Design review of the part built by this model. Coordinates are the model's own, in mm. A direction names the side the tool comes from. Coordinates: 2 decimals unless noted, no trailing zeros. Loops run counter-clockwise (first coordinate to the right, second up) from the corner with the lowest first, then second, coordinate; pieces in that order, holes last.
Autodesk Inventor part; units mm, degrees
ref_plane "YZ Plane" through (0, 0, 0) normal (1, 0, 0) x (0, 1, 0)
ref_plane "XZ Plane" through (0, 0, 0) normal (0, 1, 0) x (-1, 0, 0)
ref_plane "XY Plane" through (0, 0, 0) normal (0, 0, 1) x (1, 0, 0)
sketch "Sketch1" plane through (0, 0, 0) normal (0, 0, 1) x (1, 0, 0)
  line L0 (0, 0) -> (0, -50.8)
  line L1 (0, -50.8) -> (4, -50.8)
  line L2 (4, 0) -> (4, -50.8)
  line L3 (0, 0) -> (4, 0)
  line L4 (0, -63.5) -> (0, -72.2)
  line L5 (0, -72.2) -> (4, -72.2)
  line L6 (4, -63.5) -> (4, -72.2)
  line L7 (0, -63.5) -> (4, -63.5)
  line L8 (0, 21.4) -> (0, 12.7)
  line L9 (0, 12.7) -> (4, 12.7)
  line L10 (4, 21.4) -> (4, 12.7)
  line L11 (0, 21.4) -> (4, 21.4)
  line L12 (44.45, 25.4) -> (57.15, 25.4)
  line L13 (44.45, 25.4) -> (44.45, 21.4)
  line L14 (44.45, 21.4) -> (57.15, 21.4)
  line L15 (57.15, 25.4) -> (57.15, 21.4)
  line L16 (44.45, -76.2) -> (57.15, -76.2)
  line L17 (57.15, -76.2) -> (57.15, -72.2)
  line L18 (44.45, -72.2) -> (57.15, -72.2)
  line L19 (44.45, -76.2) -> (44.45, -72.2)
  line L20 (101.6, 21.4) -> (4, 21.4)
  line L21 (4, 21.4) -> (4, -72.2)
  line L22 (4, -72.2) -> (101.6, -72.2)
  line L23 (101.6, -72.2) -> (101.6, 21.4)
  line L24 (50.8, 21.4) -> (50.8, -72.2)
  line L25 (101.6, 0) -> (101.6, -50.8)
  line L26 (101.6, -50.8) -> (97.6, -50.8)
  line L27 (97.6, 0) -> (97.6, -50.8)
  line L28 (101.6, 0) -> (97.6, 0)
  line L29 (101.6, -63.5) -> (101.6, -72.2)
  line L30 (101.6, -72.2) -> (97.6, -72.2)
  line L31 (97.6, -63.5) -> (97.6, -72.2)
  line L32 (101.6, -63.5) -> (97.6, -63.5)
  line L33 (101.6, 21.4) -> (101.6, 12.7)
  line L34 (101.6, 12.7) -> (97.6, 12.7)
  line L35 (101.6, 21.4) -> (97.6, 21.4)
  line L36 (97.6, 12.7) -> (97.6, 21.4)
  line L37 (97.6, 12.7) -> (97.6, 0)
  line L38 (97.6, -50.8) -> (97.6, -63.5)
extrude "Extrusion1" add sketch "Sketch1" along normal blind 4 contours L3 L2 L1 L0 | L21 L10 L20 L14 L24 L18 L22 L6 L2 | L9 L8 L11 L10 | L6 L5 L4 L7 | L13 L12 L15 L14 | L18 L17 L16 L19 | L14 L20 L36 L37 L27 L38 L31 L22 L18 L24 | L20 L23 L34 L36 | L31 L32 L23 L22 | L28 L23 L26 L27
ref_plane "Work Plane1" through (50.8, -50.8, 0) normal (1, 0, 0) x (0, 0, -1)
sketch "Sketch2" plane through (0, 0, 4) normal (0, 0, 1) x (1, 0, 0)
  circle A0 centre (10.35, 6.35) radius 1.905
  line L0 (4, 12.7) -> (4, 0)
  point P0 (0, 0)
  point P1 (4, 6.35)
  point P2 (4, 6.35)
  dimension "d2" = 3.81
  dimension "d3" = 6.35
extrude "Extrusion2" cut sketch "Sketch2" against normal through all
properties part number "Left Panel" material "Wood (Cherry)"
Q1. For line 1 (Y direction, x = 10.35, z = 0.8) (3 decimals); line 2 (Y direction, x = 88, z = 3.85); line 3 (Y direction, x = 12, z = 3.7), list the stretches that pass through material, from the lowest coordinate up.
Q2. Take a section at D-D, the plane x = 38.5. Write out the cut boundary in (y, z), then the cut area to 3 significant figures.
Q3. Clearance check with flat-ended pins moving along their axes: pin 1 Ø1.2 at (x, z) = (99.5, 3) entering from -Y; pin 2 Ø1.2 at (y, z) = (24.5, 1.5) entering from -X; pin 3 Ø1 at (y, z) = (-38.5, 1) entering from -X; pin 4 Ø2 at (x, z) = (2.5, 1) entering from +Y. State where each tip first meets the part, or that it passes through.
Q4. Take a section at B-B, the plane x = 10.35. Write out the cut boundary in (y, z) (3 decimals).
Q5. Machinability: for faces 1 (the flat face through (79, -72.2, 2)), 2 (the flat face through (2, -50.8, 2)), 3 (the flat face through (51, 25.4, 2)), 4 (the flat face through (97.6, -57, 2)), which of the approach directions +Z, -Z, +X, -X, +Y, -Y give a long, thin tool a straight path to every point of the face, cutting with its end or side? Answer none if there is none.
Q6. The part is to be moulded in two halves that separate along Y. For faces 5 (the flat face through (50, -25, 4)), 6 (the flat face through (97.6, 6, 2)), 7 (the flat face through (23, 21.4, 2)), say which applies: pulls with the +Y half, pulls with the -Y half, needs draft (parallel to the pull), parting line crosses it, or undercut.
Q7. Take a section at A-A, the plane y = 6.35. Write out the cut boundary in (x, z) (3 decimals), then the cut area to 3 significant figures.
Entries:
1. line 1: y = -72.2 to 4.445, 8.255 to 21.4
1. line 2: y = -72.2 to 21.4
1. line 3: y = -72.2 to 5.4, 7.3 to 21.4
2. outline: (-72.2, 0) - (21.4, 0) - (21.4, 4) - (-72.2, 4) - close
2. area: 374 mm2
3. pin 1: stops at y = -72.2
3. pin 2: stops at x = 44.45
3. pin 3: stops at x = 0
3. pin 4: stops at y = 21.4
4. outline: (-72.2, 0) - (4.445, 0) - (4.445, 4) - (-72.2, 4) - close; (8.255, 0) - (21.4, 0) - (21.4, 4) - (8.255, 4) - close
5. face 1: +Z, -Z, +X, -Y
5. face 2: +Z, -Z, -X
5. face 3: +Z, -Z, +X, -X, +Y
5. face 4: +Z, -Z, +X
6. face 5: needs draft
6. face 6: undercut
6. face 7: pulls with the +Y half
7. outline: (4, 0) - (8.445, 0) - (8.445, 4) - (4, 4) - close; (12.255, 0) - (97.6, 0) - (97.6, 4) - (12.255, 4) - close
7. area: 359 mm2
